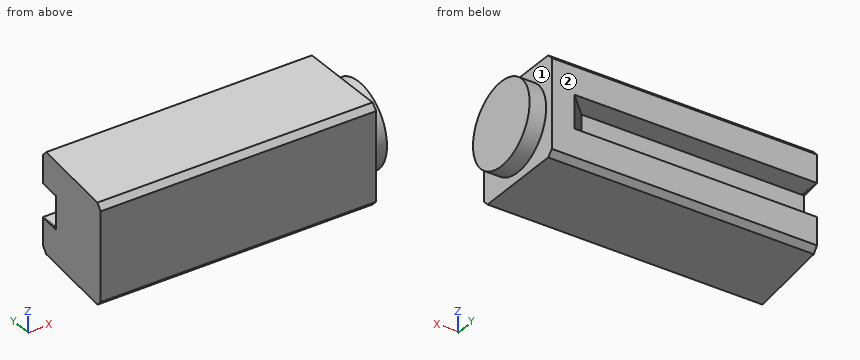
from build123d import *

# Parameters (mm, degrees)
SKETCH1_W           = 12.2174
SKETCH1_H           = 4.5847
BOSS_EXTRUDE1_DEPTH = 4.5847
SKETCH2_W           = 11.176
SKETCH2_H           = 1.524
CUT_EXTRUDE1_DEPTH  = 1.016
SKETCH4_W           = 1.524
SKETCH4_H           = 1.016
CUT_EXTRUDE3_DEPTH  = 14.249120928
SKETCH5_R           = 1.905
BOSS_EXTRUDE3_DEPTH = 0.762
CHAMFER1_SIZE       = 0.254
BOSS_EXTRUDE4_REACH = 9.861


with BuildPart() as part:
    # Sketch1 → Boss-Extrude1 (new body)
    with BuildSketch(Plane.XY):
        Polygon((-6.1087, 2.29235), (-6.5913, -2.29235), (-6.1087, -2.29235), align=None)
        Rectangle(SKETCH1_W, SKETCH1_H)
    extrude(amount=BOSS_EXTRUDE1_DEPTH)

    # Sketch2 → Cut-Extrude1 (cut)
    with BuildSketch(Plane(origin=(0, 2.29235, 0), x_dir=(1, 0, 0), z_dir=(0, 1, 0))):
        with Locations((-0.5207, -2.29235)):
            Rectangle(SKETCH2_W, SKETCH2_H)
    extrude(amount=-CUT_EXTRUDE1_DEPTH, mode=Mode.SUBTRACT)

    # Sketch4 → Cut-Extrude3 (cut, through all)
    with BuildSketch(Plane(origin=(-6.1087, 0, 0), x_dir=(0, 0, -1), z_dir=(1, 0, 0))):
        with Locations((-2.286, 1.78435)):
            Rectangle(SKETCH4_W, SKETCH4_H)
    extrude(amount=-CUT_EXTRUDE3_DEPTH, mode=Mode.SUBTRACT)

    # Sketch5 → Boss-Extrude3 (add)
    with BuildSketch(Plane(origin=(6.1087, 0, 0), x_dir=(0, 0, -1), z_dir=(1, 0, 0))):
        with Locations(Location((-2.29235, 0, 0), (0, 0, 180))):
            Circle(SKETCH5_R)
    extrude(amount=BOSS_EXTRUDE3_DEPTH)

    # Chamfer1
    chamfer1_edges = [part.edges().sort_by_distance(p)[0] for p in [
        (-0.2413, -2.29235, 4.5847),
        (0, 2.29235, 4.5847),
        (0, 2.29235, 0),
        (-0.2413, -2.29235, 0),
    ]]
    chamfer(chamfer1_edges, length=CHAMFER1_SIZE)

    # Sketch6 → Boss-Extrude4 (add, up to next)
    with BuildSketch(Plane.XY.offset(1.53035), mode=Mode.PRIVATE) as boss_extrude4_sk1:
        Polygon((5.0673, 2.29235), (5.0673, 1.27635), (4.0513, 1.27635), align=None)
    boss_extrude4_tool1 = extrude(boss_extrude4_sk1.sketch, amount=BOSS_EXTRUDE4_REACH, mode=Mode.PRIVATE) - part.part
    add(boss_extrude4_tool1.solids().sort_by_distance((4.728633, 1.615017, 1.53035))[0])


solid = part.part
Source: CAD feature listing. Evaluate the final solid. Frame: model axes, mm. Face numbers are marked on the shaded views. A direction names the side the tool comes from. Give positions to 0.01 mm unless a question says otherwise; leave off trailing zeros. Write each loop counter-clockwise with the first axis right and the second up, starting at its lowest first coordinate (ties: lowest second). Pieces come first, ordered by that corner, then holes. Notation, with made-up numbers: (10, 34) -> (20, 34) arc R33 ccw to (20, 63) -> close; hole circle Ø4 at (24.25, 9). An arc over 180 degrees is marked (long way). Return JSON: item names as keys, results as strings. Group by question number.
1. Section D-D, the plane z = 2.9. Output: boundary loops of the cut face in (x, y), then the cut area to 3 significant figures.
2. Section B-B, the plane y = 0. Output: boundary loops of the cut face in (x, z).
3. Access query for the marked faces 1 and 2. Directions: +Z, -Z, +X, -X, +Y, -Y. A direction counts if a zero-diameter tool reaches every point of the face in a straight line with its end or side. Return the directions, or none.
4. Pin query (flat end, axial travel): pin 1 Ø1 at (x, z) = (-4.5, 2.5) entering from +Y. Return the tip coordinate at first contact, or that it passes through.
5. Section C-C, the plane z = 1.4. Output: boundary loops of the cut face in (x, y), then the cut area to 3 significant figures.
6. Section A-A, the plane x = 3.25. Output: boundary loops of the cut face in (y, z), then the cut area to 3 significant figures.
7. Material intervals for line 1 (Z direction, x = 4.25, y = 1.55); line 2 (Y direction, x = 0, z = 2.9); line 3 (Z direction, x = -1, y = 2.1), sorted ascending. Write a range as from..to.
Determined:
{
 "1": {"outline": "(-6.59, -2.29) -> (6.11, -2.29) -> (6.11, -1.81) -> (6.87, -1.81) -> (6.87, 1.81) -> (6.11, 1.81) -> (6.11, 2.29) -> (5.07, 2.29) -> (4.05, 1.28) -> (-6.22, 1.28) -> close", "area": "49.0 mm2"},
 "2": {"outline": "(-6.35, 0) -> (6.11, 0) -> (6.11, 0.39) -> (6.87, 0.39) -> (6.87, 4.2) -> (6.11, 4.2) -> (6.11, 4.58) -> (-6.35, 4.58) -> close"},
 "3": {"face 1": "+X", "face 2": "+Z, -Z, +X, -X, +Y"},
 "4": {"pin 1": "stops at y = 1.28"},
 "5": {"outline": "(-6.59, -2.29) -> (6.11, -2.29) -> (6.11, -1.68) -> (6.87, -1.68) -> (6.87, 1.68) -> (6.11, 1.68) -> (6.11, 2.29) -> (-6.11, 2.29) -> close", "area": "59.7 mm2"},
 "6": {"outline": "(-2.29, 0.25) -> (-2.04, 0) -> (2.04, 0) -> (2.29, 0.25) -> (2.29, 1.53) -> (1.28, 1.53) -> (1.28, 3.05) -> (2.29, 3.05) -> (2.29, 4.33) -> (2.04, 4.58) -> (-2.04, 4.58) -> (-2.29, 4.33) -> close", "area": "19.3 mm2"},
 "7": {"line 1": "z = 0..1.53, 3.05..4.58", "line 2": "y = -2.29..1.28", "line 3": "z = 0.06..1.53, 3.05..4.52"}
}
